```python
from build123d import *

# Parameters (mm, degrees)
F0_R     = 13.49375
F1_DEPTH = 31.75
F3_D     = 22.225
F4_R     = 13.5255
F5_DEPTH = 31.75
F7_D     = 22.225
F7_DEPTH = 31.75


with BuildPart() as f1:
    # F0 (on Right) → F1 (new body, symmetric)
    with BuildSketch(Plane.YZ):
        Circle(F0_R)
    extrude(amount=F1_DEPTH, both=True)

    # F3 (through all)
    with Locations(Plane.YZ.offset(31.75)):
        with Locations((0, 0)):
            Hole(F3_D / 2)

    # F4 (on Top) → F5 (join)
    with BuildSketch(Plane.XY):
        Circle(F4_R)
    extrude(amount=F5_DEPTH)

    # F7
    with Locations(Plane.XY.offset(31.75)):
        with Locations((0, 0)):
            Hole(F7_D / 2, depth=F7_DEPTH)


solid = f1.part
```
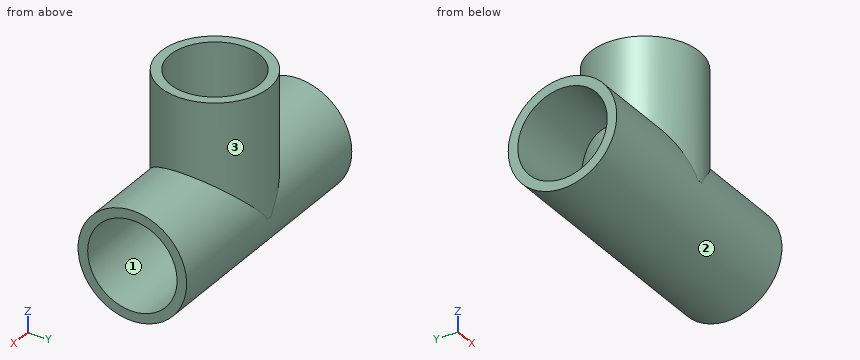
Input: part model. Units: mm. Frame: model coordinates. Face numbers are marked on the shaded views. Give positions to 0.01 mm unless a question says otherwise; leave off trailing zeros. Order: outer loops, then holes, each group sorted by start corner. A loop starts at its lowest first (then second) coordinate and runs counter-clockwise, first axis right, second up.
1. Material intervals for L1, parallel to Z at x = -23.5, y = 0.5; L2, parallel to Y at x = 3, z = 10.5, sorted ascending.
Derived:
L1: z = -13.48 to -11.1, 11.1 to 13.48
L2: y = -13.19 to -10.7, 10.7 to 13.19
2. Pin query (flat end, axial travel): pin 1 (2 mm diameter, centred on x = 13, z = 18.5, fed in from -Y); pin 2 (10 mm diameter, centred on x = -12.5, y = 9, fed in from -Z); pin 3 (5 mm diameter, centred on x = -17.5, y = 4, fed in from -Z). Return the tip coordinate at first contact, or that it passes through.
Derived:
pin 1: stops at y = -6.24
pin 2: stops at z = -12.89
pin 3: stops at z = -13.41
3. Mould query, pull axis Z, two halves, no side actions, for the marked faces 1, 2 and 3. Classes: released by +Z, released by -Z, zero draft, split by the parting line, or undercut.
Derived:
face 1: undercut
face 2: split by the parting line
face 3: zero draft
4. Section B-B on x = -17.5. Return the cut outline in (y, z) (1 decimal), and give its area (3 significant figures).
Derived:
outline: circle Ø27 at (0, 0); hole circle Ø22.2 at (0, 0)
area: 184 mm2
5. Section A-A on y = 0. Return the cut outline in (x, z).
Derived:
outline: (-31.75, -13.49) - (31.75, -13.49) - (31.75, -11.11) - (-31.75, -11.11) - close; (-31.75, 11.11) - (-13.53, 11.11) - (-13.53, 0) - (-11.11, 0) - (-11.11, 31.75) - (-13.53, 31.75) - (-13.53, 13.49) - (-31.75, 13.49) - close; (11.11, 0) - (13.53, 0) - (13.53, 11.11) - (31.75, 11.11) - (31.75, 13.49) - (13.53, 13.49) - (13.53, 31.75) - (11.11, 31.75) - close
